Verification items for the finished model (mm, model axes). Face numbers are marked on the shaded views. A direction names the side the tool comes from. Round coordinates to 2 decimals unless told otherwise and drop trailing zeros. Order: outer loops, then holes, each group sorted by start corner. A loop starts at its lowest first (then second) coordinate and runs counter-clockwise, first axis right, second up. Notation, with made-up numbers: M -8.5,-34 L 47.5,-34 A27 cw 47.5,-17 Z; hole C 57,65.5 d1. An arc over 180 degrees is marked long. Use CSV: the item, a comma, the result in double quotes. Start each with the question number.
Q1. Mould release check, pull along X, two halves, no side actions. Record for the marked faces 3, 4, 5 and 6: +X half, -X half, draft (parallel to the pull), parting line (faces both ways), or undercut.
Q2. Scan lines: line 1 (Y direction, x = 0, z = -1.25); line 2 (Z direction, x = -7, y = -18); line 3 (Y direction, x = -3, z = -3.25). Record each from-to range of solid material in increasing order.
Q3. Sectioned sample at A-A (x = 0). Enter the section's corners in (y, z), and give its area (3 significant figures).
Q4. Set-up check for the marked faces 1 and 2: record each of +Z, -Z, +X, -X, +Y, -Y from which the full face is reachable in a straight line by a thin tool's end or side.
Q5. Sectioned sample at C-C (z = -4.5). Enter the section's corners in (x, y).
Q6. Gauge pin test, flat ends, axial feed: pin 1 Ø0.9 at (x, z) = (-13.5, -6.5) entering from +Y; pin 2 Ø1 at (y, z) = (-7, -6.5) entering from +X; pin 3 Ø12.5 at (x, y) = (-5.5, -12) entering from -Z; pin 4 Ø1 at (y, z) = (-7.5, -6) entering from -X. Record the tip position at first contact, or that the pin passes through.
Q7. Sectioned sample at D-D (y = -7). Enter the section's corners in (x, z).
Q8. Sectioned sample at B-B (y = -15). Enter the section's corners in (x, z), and give its area (3 significant figures).
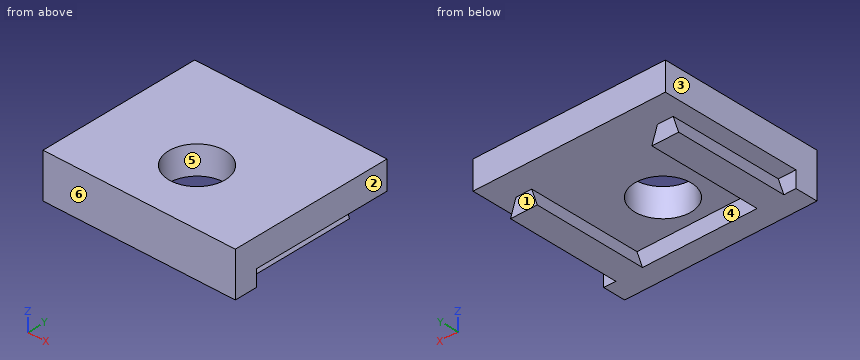
```python
from build123d import *
from OCP.BRepFilletAPI import BRepFilletAPI_MakeChamfer

# Parameters (mm, degrees)
SKETCH_1_R          = 5
EXTRUDE_1_DEPTH     = 5
EXTRUDE_2_REACH     = 42.012
EXTRUDE_3_DEPTH     = 55
EXTRUDE_4_DEPTH     = 20
FILLET_1_R          = 10
CHAMFER_1_SIZE      = 1
CHAMFER_1_SIZE2     = 1.741048535
CHAMFER_1_SIZE2_2   = 3.661578825
CHAMFER_1_SIZE2_3   = 2.732050808
CUT_EXTRUDE_1_REACH = 86.876
SKETCH_5_R          = 1.65
SKETCH_6_R          = 54.70604167
CUT_EXTRUDE_2_DEPTH = 66.501221402
SKETCH_7_W          = 77.77608505
SKETCH_7_H          = 88.124851988
SKETCH_7_W_2        = 34.010032192
SKETCH_7_H_2        = 31.175862843
CUT_EXTRUDE_3_DEPTH = 41.477277576


with BuildPart() as part:
    # 草图1 → 凸台-拉伸1 (new body)
    with BuildSketch(Plane.XY):
        Polygon((-20, 26), (20, 26), (30, 0), (20, -26), (-20, -26), (-30, 0), align=None)
        with Locations((0, -15)):
            Circle(SKETCH_1_R, mode=Mode.SUBTRACT)
    extrude(amount=-EXTRUDE_1_DEPTH)

    # 凸台-拉伸2: up to this plane
    extrude_2_end = Plane(origin=(0, 24.665063509, -42.72114317), z_dir=(0, 0.499999999999998, -0.8660254037844398))
    # 草图2 → 凸台-拉伸2 (add, up to the surface)
    with BuildSketch(Plane(origin=(0, 0, -5), x_dir=(-1, 0, 0), z_dir=(0, 0, -1)), mode=Mode.PRIVATE) as extrude_2_sk1:
        Polygon((-20, 26), (20, 26), (21.923076923, 21), (-21.923076923, 21), align=None)
    extrude_2_tool1 = split(extrude(extrude_2_sk1.sketch, amount=EXTRUDE_2_REACH, mode=Mode.PRIVATE), bisect_by=extrude_2_end, keep=Keep.BOTH, mode=Mode.PRIVATE)
    add(extrude_2_tool1.solids().sort_by_distance((0, 23.461774, -5))[0])

    # 草图3 → 凸台-拉伸3 (add)
    with BuildSketch(Plane(origin=(0, 0, -5), x_dir=(-1, 0, 0), z_dir=(0, 0, -1))):
        Polygon((23.846153846, -16), (20, -26), (-20, -26), (-23.846153846, -16), (-19.560495915, -16), (-17.252803607, -22), (17.252803607, -22), (19.560495915, -16), align=None)
    extrude(amount=EXTRUDE_3_DEPTH)

    # 草图4 → 凸台-拉伸4 (add)
    with BuildSketch(Plane(origin=(0, -2, 0), x_dir=(1, 0, 0), z_dir=(0, 1, 0))):
        Polygon((11.105409255, 5), (10.138742589, 7.9), (14.861257411, 7.9), (13.894590745, 5), align=None)
        Polygon((-11.105409255, 5), (-13.894590745, 5), (-14.861257411, 7.9), (-10.138742589, 7.9), align=None)
    extrude(amount=-EXTRUDE_4_DEPTH)

    # 圆角1
    fillet_1_edges = [part.edges().sort_by_distance(p)[0] for p in [
        (-21.70332488, -16, -60),
        (21.70332488, -16, -5),
        (-21.70332488, -16, -5),
        (-20.961538462, 23.5, -43.393792901),
        (20.961538462, 23.5, -43.393792901),
    ]]
    fillet(fillet_1_edges, radius=FILLET_1_R - 0.0001)  # a hair under: the kernel refuses the full size

    # 倒角1: one chamfer whose edges measure the first distance from different faces: ONE call of the kernel's chamfer builder (chamfer() names one face for all edges)
    chamfer_1_edges_1 = [part.edges().sort_by_distance(p)[0] for p in [
        (20, 26, -16.238036635),
    ]]
    chamfer_1_side_1 = [part.faces().sort_by_distance(p)[0] for p in [
        (20.161601575, 25.579835904, -16.238036635),
    ]]
    chamfer_1_edges_2 = [part.edges().sort_by_distance(p)[0] for p in [
        (17.633378474, 26, -39.139308282),
        (-17.633378474, 26, -39.139308282),
    ]]
    chamfer_1_side_2 = [part.faces().sort_by_distance(p)[0] for p in [
        (0, 26, -20.586375743),
    ]]
    chamfer_1_edges_3 = [part.edges().sort_by_distance(p)[0] for p in [
        (0, 26, -41.950417228),
    ]]
    chamfer_1_side_3 = [part.faces().sort_by_distance(p)[0] for p in [
        (0, 26, -20.586375743),
    ]]
    chamfer_1_edges_4 = [part.edges().sort_by_distance(p)[0] for p in [
        (-20, 26, -16.238036635),
    ]]
    chamfer_1_side_4 = [part.faces().sort_by_distance(p)[0] for p in [
        (-21.761475348, 21.420164096, -20.181412308),
    ]]
    chamfer_1 = BRepFilletAPI_MakeChamfer(part.part.solid().wrapped)
    for e in chamfer_1_edges_1:
        chamfer_1.Add(CHAMFER_1_SIZE, CHAMFER_1_SIZE2, e.wrapped, chamfer_1_side_1[0].wrapped)  # the first distance lies on this face
    for e in chamfer_1_edges_2:
        chamfer_1.Add(CHAMFER_1_SIZE, CHAMFER_1_SIZE2_2, e.wrapped, chamfer_1_side_2[0].wrapped)  # the first distance lies on this face
    for e in chamfer_1_edges_3:
        chamfer_1.Add(CHAMFER_1_SIZE, CHAMFER_1_SIZE2_3, e.wrapped, chamfer_1_side_3[0].wrapped)  # the first distance lies on this face
    for e in chamfer_1_edges_4:
        chamfer_1.Add(CHAMFER_1_SIZE, CHAMFER_1_SIZE2, e.wrapped, chamfer_1_side_4[0].wrapped)  # the first distance lies on this face
    add(Compound.cast(chamfer_1.Shape()), mode=Mode.REPLACE)

    # 草图5 → 切除-拉伸1 (cut, up to next)
    with BuildSketch(Plane(origin=(0, 26, 0), x_dir=(1, 0, 0), z_dir=(0, 1, 0)), mode=Mode.PRIVATE) as cut_extrude_1_sk1:
        with Locations((14, 36)):
            Circle(SKETCH_5_R)
    cut_extrude_1_tool1 = extrude(cut_extrude_1_sk1.sketch, amount=-CUT_EXTRUDE_1_REACH, mode=Mode.PRIVATE) & part.part
    # 草图5 → 切除-拉伸1 (cut, up to next)
    with BuildSketch(Plane(origin=(0, 26, 0), x_dir=(1, 0, 0), z_dir=(0, 1, 0)), mode=Mode.PRIVATE) as cut_extrude_1_sk2:
        with Locations((14, 8)):
            Circle(SKETCH_5_R)
    cut_extrude_1_tool2 = extrude(cut_extrude_1_sk2.sketch, amount=-CUT_EXTRUDE_1_REACH, mode=Mode.PRIVATE) & part.part
    # 草图5 → 切除-拉伸1 (cut, up to next)
    with BuildSketch(Plane(origin=(0, 26, 0), x_dir=(1, 0, 0), z_dir=(0, 1, 0)), mode=Mode.PRIVATE) as cut_extrude_1_sk3:
        with Locations((-14, 8)):
            Circle(SKETCH_5_R)
    cut_extrude_1_tool3 = extrude(cut_extrude_1_sk3.sketch, amount=-CUT_EXTRUDE_1_REACH, mode=Mode.PRIVATE) & part.part
    # 草图5 → 切除-拉伸1 (cut, up to next)
    with BuildSketch(Plane(origin=(0, 26, 0), x_dir=(1, 0, 0), z_dir=(0, 1, 0)), mode=Mode.PRIVATE) as cut_extrude_1_sk4:
        with Locations((-14, 36)):
            Circle(SKETCH_5_R)
    cut_extrude_1_tool4 = extrude(cut_extrude_1_sk4.sketch, amount=-CUT_EXTRUDE_1_REACH, mode=Mode.PRIVATE) & part.part
    # 草图5 → 切除-拉伸1 (cut, up to next)
    with BuildSketch(Plane(origin=(0, 26, 0), x_dir=(1, 0, 0), z_dir=(0, 1, 0)), mode=Mode.PRIVATE) as cut_extrude_1_sk5:
        with Locations((10, 22)):
            Circle(SKETCH_5_R)
    cut_extrude_1_tool5 = extrude(cut_extrude_1_sk5.sketch, amount=-CUT_EXTRUDE_1_REACH, mode=Mode.PRIVATE) & part.part
    # 草图5 → 切除-拉伸1 (cut, up to next)
    with BuildSketch(Plane(origin=(0, 26, 0), x_dir=(1, 0, 0), z_dir=(0, 1, 0)), mode=Mode.PRIVATE) as cut_extrude_1_sk6:
        with Locations((-10, 22)):
            Circle(SKETCH_5_R)
    cut_extrude_1_tool6 = extrude(cut_extrude_1_sk6.sketch, amount=-CUT_EXTRUDE_1_REACH, mode=Mode.PRIVATE) & part.part
    # 草图5 → 切除-拉伸1 (cut, up to next)
    with BuildSketch(Plane(origin=(0, 26, 0), x_dir=(1, 0, 0), z_dir=(0, 1, 0)), mode=Mode.PRIVATE) as cut_extrude_1_sk7:
        with Locations((0, 12)):
            Circle(SKETCH_5_R)
    cut_extrude_1_tool7 = extrude(cut_extrude_1_sk7.sketch, amount=-CUT_EXTRUDE_1_REACH, mode=Mode.PRIVATE) & part.part
    # 草图5 → 切除-拉伸1 (cut, up to next)
    with BuildSketch(Plane(origin=(0, 26, 0), x_dir=(1, 0, 0), z_dir=(0, 1, 0)), mode=Mode.PRIVATE) as cut_extrude_1_sk8:
        with Locations((0, 32)):
            Circle(SKETCH_5_R)
    cut_extrude_1_tool8 = extrude(cut_extrude_1_sk8.sketch, amount=-CUT_EXTRUDE_1_REACH, mode=Mode.PRIVATE) & part.part
    add(cut_extrude_1_tool1.solids().sort_by_distance((14, 26, -36))[0], mode=Mode.SUBTRACT)
    add(cut_extrude_1_tool2.solids().sort_by_distance((14, 26, -8))[0], mode=Mode.SUBTRACT)
    add(cut_extrude_1_tool3.solids().sort_by_distance((-14, 26, -8))[0], mode=Mode.SUBTRACT)
    add(cut_extrude_1_tool4.solids().sort_by_distance((-14, 26, -36))[0], mode=Mode.SUBTRACT)
    add(cut_extrude_1_tool5.solids().sort_by_distance((10, 26, -22))[0], mode=Mode.SUBTRACT)
    add(cut_extrude_1_tool6.solids().sort_by_distance((-10, 26, -22))[0], mode=Mode.SUBTRACT)
    add(cut_extrude_1_tool7.solids().sort_by_distance((0, 26, -12))[0], mode=Mode.SUBTRACT)
    add(cut_extrude_1_tool8.solids().sort_by_distance((0, 26, -32))[0], mode=Mode.SUBTRACT)

    # 草图6 → 切除-拉伸2 (cut, through all)
    with BuildSketch(Plane(origin=(0, 0, -7.9), x_dir=(-1, 0, 0), z_dir=(0, 0, -1))):
        with Locations((0, -15)):
            Circle(SKETCH_6_R)
    extrude(amount=CUT_EXTRUDE_2_DEPTH, mode=Mode.SUBTRACT)

    # 草图7 → 切除-拉伸3 (cut, through all)
    with BuildSketch(Plane(origin=(0, 0, -7.9), x_dir=(-1, 0, 0), z_dir=(0, 0, -1))):
        with Locations((0, -12.753762072)):
            Rectangle(SKETCH_7_W, SKETCH_7_H)
        with Locations((0, -12.753762073)):
            Rectangle(SKETCH_7_W_2, SKETCH_7_H_2, mode=Mode.SUBTRACT)
    extrude(amount=-CUT_EXTRUDE_3_DEPTH, mode=Mode.SUBTRACT)


solid = part.part
```
Verdict:
1,face 3,"-X half"
1,face 4,"undercut"
1,face 5,"undercut"
1,face 6,"draft"
2,line 1,"y = -26 to -20, -10 to 2.83"
2,line 2,"z = -5 to 0"
2,line 3,"y = -26 to -19, -11 to 2.83"
3,outline,"M -26,-7.9 L -22,-7.9 L -22,-5 L -20,-5 L -20,0 L -26,0 Z; M -10,-5 L 2.83,-5 L 2.83,0 L -10,0 Z"
3,area,"106 mm²"
4,face 1,"-Z, +X, -X, +Y"
4,face 2,"+Z, -Z, +X, +Y, -Y"
5,outline,"M -17.01,-26 L 17.01,-26 L 17.01,2.83 L -17.01,2.83 Z; hole C 0,-15 d10"
6,pin 1,"stops at y = -2"
6,pin 2,"stops at x = 14.56"
6,pin 3,"stops at z = -7.9"
6,pin 4,"stops at x = -14.39"
7,outline,"M -17.01,-5 L -13.89,-5 L -14.86,-7.9 L -10.14,-7.9 L -11.11,-5 L 11.11,-5 L 10.14,-7.9 L 14.86,-7.9 L 13.89,-5 L 17.01,-5 L 17.01,0 L -17.01,0 Z"
8,outline,"M -17.01,-5 L -13.89,-5 L -14.86,-7.9 L -10.14,-7.9 L -11.11,-5 L -5,-5 L -5,0 L -17.01,0 Z; M 5,-5 L 11.11,-5 L 10.14,-7.9 L 14.86,-7.9 L 13.89,-5 L 17.01,-5 L 17.01,0 L 5,0 Z"
8,area,"142 mm²"
